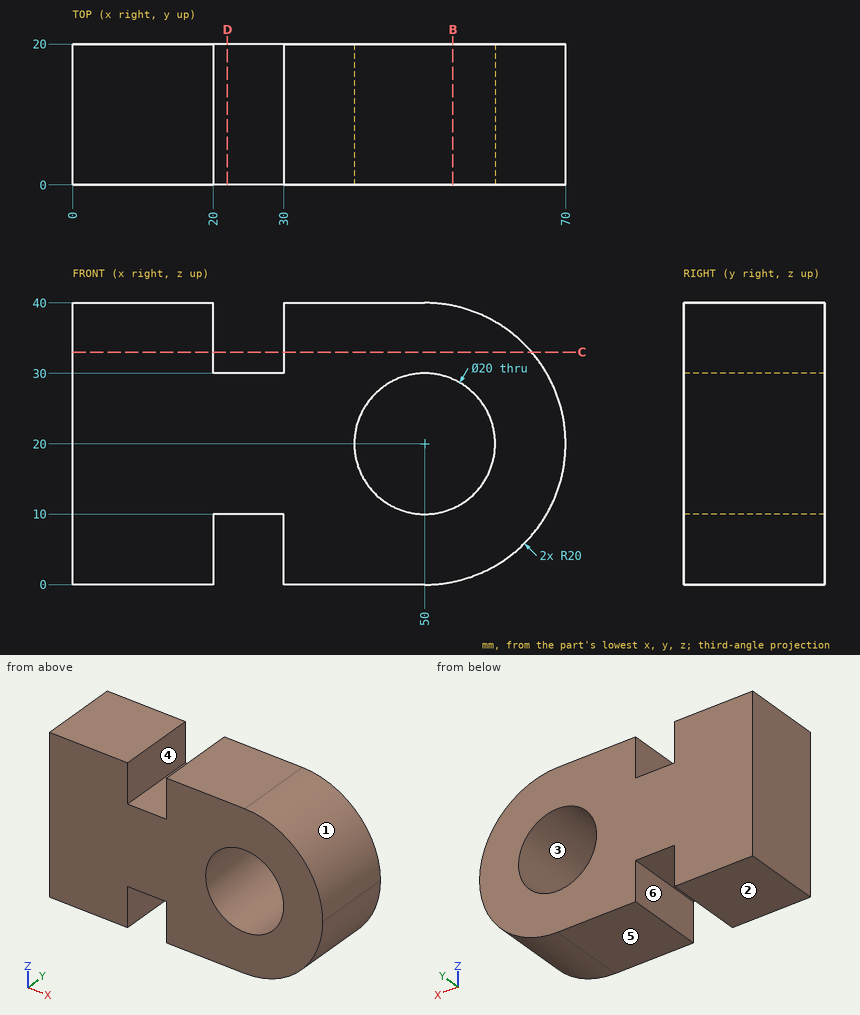
Can you work these out from the drawing? Everything is in mm from the part's minimum corner. A direction names the side the tool comes from. Give positions to 0.01 mm unless a question says otherwise; leave off trailing zeros. Loops run counter-clockwise (first coordinate to the right, second up) from the corner with the lowest first, then second, coordinate; pieces in that order, holes last. Notation, with made-up numbers: (-13.75, -32.5) -> (22.25, -32.5) arc R31 ccw to (22.25, -5.5) -> close; hole circle Ø3 at (66, -18). An arc over 180 degrees is marked (long way). Write item = value, one per line.
1) I need wall thicknesses on L1, parallel to X at y = 8, z = 20; L2, parallel to Z at x = 50, y = 10; L3, parallel to Z at x = 25, y = 7. Which ranges of each line are inside material? Lowest first, please. Write a range as from..to.
Check result:
L1 = 0..40, 60..70
L2 = 0..10, 30..40
L3 = 10..30
2) For the marked faces 4, 5 and 6, which set-ups out of +Z, -Z, +X, -X, +Y, -Y let a thin tool reach every point of the face, with its end or its side?
Check result:
face_4 = +Z, +Y, -Y
face_5 = -Z, +X, -X, +Y, -Y
face_6 = -Z, +Y, -Y
3) Will these pins go through, and if not, where does the flat tip stop? pin 1 (3 mm diameter, centred on y = 8.5, z = 34, fed in from +X); pin 2 (1.5 mm diameter, centred on x = 22.5, y = 5.5, fed in from +Z); pin 3 (8 mm diameter, centred on y = 12.5, z = 7, fed in from +X).
Check result:
pin_1 = 65.61
pin_2 = 30
pin_3 = 67.86
4) Suppose I cut it at B-B on x = 54. Write out the boundary of the cut face in (y, z) (3 decimals), then the cut area to 3 significant figures.
Check result:
outline = (0, 0.404) -> (20, 0.404) -> (20, 10.835) -> (0, 10.835) -> close; (0, 29.165) -> (20, 29.165) -> (20, 39.596) -> (0, 39.596) -> close
area = 417 mm2
5) Thinking about a two-plate mould opening in Z: for the marked faces 1, 2 and 3, which applies, released by +Z, released by -Z, zero draft, split by the parting line, or undercut?
Check result:
face_1 = released by +Z
face_2 = released by -Z
face_3 = undercut
6) Suppose I cut it at C-C on z = 33. Write out the boundary of the cut face in (x, y).
Check result:
outline = (0, 0) -> (20, 0) -> (20, 20) -> (0, 20) -> close; (30, 0) -> (65.2, 0) -> (65.2, 20) -> (30, 20) -> close
7) Suppose I cut it at D-D on x = 22. Write out the boundary of the cut face in (y, z).
Check result:
outline = (0, 10) -> (20, 10) -> (20, 30) -> (0, 30) -> close
